For this review, take the finished solid that the model builds, in its own axes (mm). Face numbers are marked on the shaded views. A direction names the side the tool comes from. Coordinates: 2 decimals unless noted, no trailing zeros. Loops run counter-clockwise (first coordinate to the right, second up) from the corner with the lowest first, then second, coordinate; pieces in that order, holes last. Notation, with made-up numbers: M 32.25,65.5 L 75.25,65.5 A20 cw 75.25,87.5 Z; hole C 74,18 d4. An arc over 180 degrees is marked long. Answer as a JSON object with one key per item and string values. Group by question number.
Item 1: Wall thickness on L1, parallel to Y at x = 2.5, z = 8.5; L2, parallel to Z at x = 0, y = 27; L3, parallel to X at y = 103.5, z = 13: over which ranges is each line inside the solid? List them lowest first. Write a range as from..to.
Item 2: Insertion check: pin 1 (4 mm diameter, centred on y = 91.5, z = 7, fed in from +X); pin 2 (10 mm diameter, centred on y = 73, z = -7, fed in from -X); pin 3 (12 mm diameter, centred on y = 46.5, z = 6.5, fed in from +X). Each pin has a flat end and moves straight along its axis. Give the tip position at first contact, or say it passes through.
Item 3: Tool access review of the marked faces 1 and 2: name each direction out of +Z, -Z, +X, -X, +Y, -Y from which nothing blocks a thin tool from reaching the whole face with its end or side.
Item 4: Mouldability with a two-part tool opening along X and no side actions: class the marked faces 3, 4 and 5 as +X half, -X half, draft (parallel to the pull), parting line (faces both ways), or undercut.
Item 5: Add section C-C (y = 24). State the section outline as (x, z) points, then the cut area to 3 significant figures.
Item 6: Add section D-D (x = 9.5). State the section outline as (y, z) points, then the cut area to 3 significant figures.
Item 7: Add section A-A (z = -19). State the section outline as (x, y) points.
Item 8: Add section B-B (x = 14.5). State the section outline as (y, z) points.
from build123d import *

# Parameters (mm, degrees)
SKETCH1_R            = 24.13
BOSS_EXTRUDE1_DEPTH  = 109.22
CUT_EXTRUDE7_DEPTH   = 2.54
CIRPATTERN2_COUNT    = 4
MIRROR1_COPY_1_DEPTH = 2.54
MIRROR1_COPY_2_DEPTH = 2.54
MIRROR1_COPY_3_DEPTH = 2.54


with BuildPart() as part:
    # Sketch1 → Boss-Extrude1 (new body)
    with BuildSketch(Plane(origin=(0, 0, 0), x_dir=(1, 0, 0), z_dir=(0, 1, 0))):
        Circle(SKETCH1_R)
    extrude(amount=BOSS_EXTRUDE1_DEPTH)

    # Sketch2 → Cut-Extrude7 (cut)
    with BuildSketch(Plane(origin=(0, 109.22, 0), x_dir=(1, 0, 0), z_dir=(0, 1, 0))):
        with BuildLine():
            Line((-13.398366618, -20.068399836), (0.023672, -0.252894516))
            ThreePointArc((0.023672, -0.252894516), (-0.212080054, -0.139778577), (-0.223069042, 0.12147511))
            Line((-0.223069042, 0.12147511), (-23.725561751, -4.399388549))
            ThreePointArc((-23.725561751, -4.399388549), (-20.147605145, -13.278964829), (-13.398366618, -20.068399836))
        make_face()
    cut_extrude7 = extrude(amount=-CUT_EXTRUDE7_DEPTH, mode=Mode.SUBTRACT)

    # CirPattern2: Cut-Extrude7 ×4 about axis
    cirpattern2_axis = Axis((0, 0, 0), (0, 1, 0))
    for i in range(1, CIRPATTERN2_COUNT):
        add(cut_extrude7.rotate(cirpattern2_axis, i * 360 / CIRPATTERN2_COUNT), mode=Mode.SUBTRACT)

    # Mirror1: Cut-Extrude7 across plane
    add(cut_extrude7.mirror(Plane.ZX.offset(54.61)), mode=Mode.SUBTRACT)

    # Mirror1 copy 1 sketch → Mirror1 copy 1 (cut)
    with BuildSketch(Plane(origin=(0, 0, 0), x_dir=(0, 0, -1), z_dir=(0, -1, 0))):
        with BuildLine():
            Line((-13.398366618, 20.068399836), (0.023672, 0.252894516))
            ThreePointArc((0.023672, 0.252894516), (-0.212080054, 0.139778577), (-0.223069042, -0.12147511))
            Line((-0.223069042, -0.12147511), (-23.725561751, 4.399388549))
            ThreePointArc((-23.725561751, 4.399388549), (-20.147605145, 13.278964829), (-13.398366618, 20.068399836))
        make_face()
    extrude(amount=-MIRROR1_COPY_1_DEPTH, mode=Mode.SUBTRACT)

    # Mirror1 copy 2 sketch → Mirror1 copy 2 (cut)
    with BuildSketch(Plane(origin=(0, 0, 0), x_dir=(-1, 0, 0), z_dir=(0, -1, 0))):
        with BuildLine():
            Line((-13.398366618, 20.068399836), (0.023672, 0.252894516))
            ThreePointArc((0.023672, 0.252894516), (-0.212080054, 0.139778577), (-0.223069042, -0.12147511))
            Line((-0.223069042, -0.12147511), (-23.725561751, 4.399388549))
            ThreePointArc((-23.725561751, 4.399388549), (-20.147605145, 13.278964829), (-13.398366618, 20.068399836))
        make_face()
    extrude(amount=-MIRROR1_COPY_2_DEPTH, mode=Mode.SUBTRACT)

    # Mirror1 copy 3 sketch → Mirror1 copy 3 (cut)
    with BuildSketch(Plane(origin=(0, 0, 0), x_dir=(0, 0, 1), z_dir=(0, -1, 0))):
        with BuildLine():
            Line((-13.398366618, 20.068399836), (0.023672, 0.252894516))
            ThreePointArc((0.023672, 0.252894516), (-0.212080054, 0.139778577), (-0.223069042, -0.12147511))
            Line((-0.223069042, -0.12147511), (-23.725561751, 4.399388549))
            ThreePointArc((-23.725561751, 4.399388549), (-20.147605145, 13.278964829), (-13.398366618, 20.068399836))
        make_face()
    extrude(amount=-MIRROR1_COPY_3_DEPTH, mode=Mode.SUBTRACT)


solid = part.part
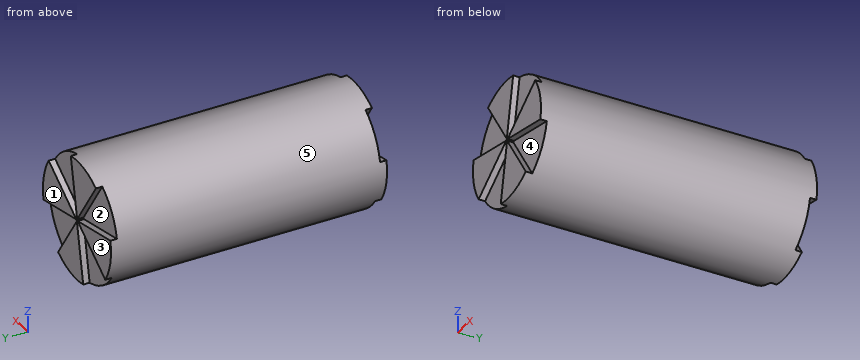
From the geometry:
{
 "1": {"L1": "y = 2.54..106.68", "L2": "z = -24.13..24.13", "L3": "x = -20.33..20.33"},
 "2": {"pin 1": "stops at x = 23.61", "pin 2": "stops at x = -24.05", "pin 3": "stops at x = 24.12"},
 "3": {"face 1": "+Z, -Z, +X, -X, +Y", "face 2": "+Y"},
 "4": {"face 3": "draft", "face 4": "undercut", "face 5": "parting line"},
 "5": {"outline": "C 0,0 d48.26", "area": "1,830 mm²"},
 "6": {"outline": "M 0,-22.18 L 109.22,-22.18 L 109.22,-14.31 L 106.68,-14.31 L 106.68,-1.66 L 109.22,-1.66 L 109.22,6.24 L 106.68,6.24 L 106.68,22.18 L 2.54,22.18 L 2.54,6.24 L 0,6.24 L 0,-1.66 L 2.54,-1.66 L 2.54,-14.31 L 0,-14.31 Z", "area": "4,700 mm²"},
 "7": {"outline": "M -14.87,2.54 L -3.49,2.54 L -3.49,0 L 12.67,0 L 12.67,2.54 L 14.87,2.54 L 14.87,106.68 L 12.67,106.68 L 12.67,109.22 L -3.49,109.22 L -3.49,106.68 L -14.87,106.68 Z"},
 "8": {"outline": "M 0,-2.62 L 2.54,-2.62 L 2.54,-19.29 L 106.68,-19.29 L 106.68,-2.62 L 109.22,-2.62 L 109.22,9.63 L 106.68,9.63 L 106.68,19.29 L 2.54,19.29 L 2.54,9.63 L 0,9.63 Z"}
}
